Part model, mm, in its own coordinate system. Face numbers are marked on the shaded views. A direction names the side the tool comes from. Give positions to 0.01 mm unless a question says otherwise; leave off trailing zeros. Loops run counter-clockwise (first coordinate to the right, second up) from the corner with the lowest first, then second, coordinate; pieces in that order, holes last. Notation, with made-up numbers: M 45,0 L 62,0 A8 cw 62,13 Z; hole C 74.25,-36 d8. An arc over 180 degrees is marked long. Answer in a Markdown table with one row per item.
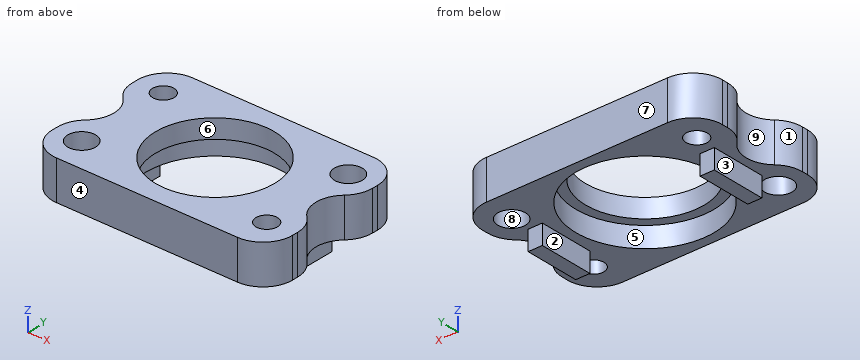
from build123d import *

# Parameters (mm, degrees)
SKETCH1_W                       = 38.735
SKETCH1_H                       = 25.4
BOSS_EXTRUDE1_DEPTH             = 6.35
CUT_EXTRUDE1_DEPTH              = 7.35
CUT_EXTRUDE2_DEPTH              = 7.35
SKETCH4_W                       = 2.286
SKETCH4_H                       = 8.89
BOSS_EXTRUDE2_DEPTH             = 3.175
SKETCH5_W                       = 2.286
SKETCH5_H                       = 8.89
BOSS_EXTRUDE3_DEPTH             = 3.175
HOLE1_D                         = 19.1262
HOLE1_DEPTH                     = 6.35
HOLE1_CBORE_D                   = 22.2758
HOLE1_CBORE_DEPTH               = 3.302
F_16_0_177_DIAMETER_HOLE1_D     = 4.4958
F_16_0_177_DIAMETER_HOLE1_DEPTH = 9.525
F_29_0_136_DIAMETER_HOLE1_D     = 3.4544
F_29_0_136_DIAMETER_HOLE1_DEPTH = 9.525
FILLET1_R                       = 4.7625


with BuildPart() as part:
    # Sketch1 → Boss-Extrude1 (new body)
    with BuildSketch(Plane.XY.offset(6.35)):
        with Locations((-234.6325, 25.4)):
            Rectangle(SKETCH1_W, SKETCH1_H)
    extrude(amount=-BOSS_EXTRUDE1_DEPTH)

    # Sketch2 → Cut-Extrude1 (cut, through all)
    with BuildSketch(Plane(origin=(0, 0, 0), x_dir=(-1, 0, 0), z_dir=(0, 0, -1))):
        with BuildLine():
            Line((215.265, 32.388210744), (215.265, 18.411789256))
            ThreePointArc((215.265, 18.411789256), (215.6632391, 20.318260617), (216.791355087, 21.905894628))
            ThreePointArc((216.791355087, 21.905894628), (218.317710174, 25.4), (216.791355087, 28.894105372))
            ThreePointArc((216.791355087, 28.894105372), (215.6632391, 30.481739383), (215.265, 32.388210744))
        make_face()
    extrude(amount=-CUT_EXTRUDE1_DEPTH, mode=Mode.SUBTRACT)

    # Sketch3 → Cut-Extrude2 (cut, through all)
    with BuildSketch(Plane(origin=(0, 0, 0), x_dir=(-1, 0, 0), z_dir=(0, 0, -1))):
        with BuildLine():
            Line((254, 20.955), (254, 29.845))
            ThreePointArc((254, 29.845), (250.969652441, 25.4), (254, 20.955))
        make_face()
    extrude(amount=-CUT_EXTRUDE2_DEPTH, mode=Mode.SUBTRACT)

    # Sketch4 → Boss-Extrude2 (add)
    with BuildSketch(Plane(origin=(0, 0, 0), x_dir=(-1, 0, 0), z_dir=(0, 0, -1))):
        with Locations((220.7641, 25.4)):
            Rectangle(SKETCH4_W, SKETCH4_H)
    extrude(amount=BOSS_EXTRUDE2_DEPTH)

    # Sketch5 → Boss-Extrude3 (add)
    with BuildSketch(Plane(origin=(0, 0, 0), x_dir=(-1, 0, 0), z_dir=(0, 0, -1))):
        with Locations((248.5009, 25.4)):
            Rectangle(SKETCH5_W, SKETCH5_H)
    extrude(amount=BOSS_EXTRUDE3_DEPTH)

    # Hole1
    with Locations(Plane(origin=(0, 0, 0), x_dir=(-1, 0, 0), z_dir=(0, 0, -1))):
        with Locations((234.6325, 25.4)):
            CounterBoreHole(HOLE1_D / 2, HOLE1_CBORE_D / 2, HOLE1_CBORE_DEPTH, depth=HOLE1_DEPTH)

    # #16 (0.177) Diameter Hole1
    with Locations(Plane.XY.offset(6.35)):
        with Locations((-249.555, 17.78), (-219.71, 33.02)):
            Hole(F_16_0_177_DIAMETER_HOLE1_D / 2, depth=F_16_0_177_DIAMETER_HOLE1_DEPTH)

    # #29 (0.136) Diameter Hole1
    with Locations(Plane.XY.offset(6.35)):
        with Locations((-219.71, 17.78), (-249.555, 33.02)):
            Hole(F_29_0_136_DIAMETER_HOLE1_D / 2, depth=F_29_0_136_DIAMETER_HOLE1_DEPTH)

    # Fillet1
    fillet1_edges = [part.edges().sort_by_distance(p)[0] for p in [
        (-254, 20.955, 3.175),
        (-254, 29.845, 3.175),
        (-254, 38.1, 3.175),
        (-215.265, 38.1, 3.175),
        (-215.265, 12.7, 3.175),
        (-254, 12.7, 3.175),
    ]]
    fillet(fillet1_edges, radius=FILLET1_R)


solid = part.part
(1) Drill centre lines: line 1 along Y through (x, z) = (-235, 3); line 2 along X through (y, z) = (27, 4.25); line 3 along Z through (x, y) = (-243.5, 35). Where is each one in solid material? Low to high.
Recorded:
| item | result |
|---|---|
| line 1 | y = 12.7 to 14.27, 36.53 to 38.1 |
| line 2 | x = -251.25 to -244.06, -225.2 to -218.04 |
| line 3 | z = 0 to 6.35 |
(2) Pin check, flat tips, straight feed: pin 1 Ø1.6 at (y, z) = (26, -1) entering from +X; pin 2 Ø1 at (y, z) = (30, 2) entering from -X; pin 3 Ø1 at (y, z) = (26, -1) entering from -X. Stop position of each tip, or through.
Recorded:
| item | result |
|---|---|
| pin 1 | stops at x = -219.62 |
| pin 2 | stops at x = -253.62 |
| pin 3 | stops at x = -249.64 |
(3) Which spindle directions (+Z, -Z, +X, -X, +Y, -Y) get a long thin tool onto all of the face, cutting with end or side? Do the marked faces 1, 2, 3, 4 and 5. Say none if no direction does.
Recorded:
| item | result |
|---|---|
| face 1 | +Z, -Z, -X |
| face 2 | -Z, +Y, -Y |
| face 3 | -Z, -X, +Y, -Y |
| face 4 | +Z, -Z, +X, -X, -Y |
| face 5 | -Z |
(4) Saw through at C-C (y = 25.4). Write the cut outline in (x, z) (3 decimals), plus the area to 3 significant figures.
Recorded:
| item | result |
|---|---|
| outline | M -250.97,0 L -249.644,0 L -249.644,-3.175 L -247.358,-3.175 L -247.358,0 L -245.77,0 L -245.77,3.302 L -244.196,3.302 L -244.196,6.35 L -250.97,6.35 Z; M -225.069,3.302 L -223.495,3.302 L -223.495,0 L -221.907,0 L -221.907,-3.175 L -219.621,-3.175 L -219.621,0 L -218.318,0 L -218.318,6.35 L -225.069,6.35 Z |
| area | 90.0 mm^2 |
(5) Pull direction X, two halves, no side cores. Call the marked faces 6, 7, 8 and 9: +X half, -X half, draft (parallel to the pull), parting line (faces both ways), or undercut.
Recorded:
| item | result |
|---|---|
| face 6 | undercut |
| face 7 | draft |
| face 8 | undercut |
| face 9 | -X half |
(6) Saw through at D-D (x = -227). Write the cut outline in (y, z), plus the area to 3 significant figures.
Recorded:
| item | result |
|---|---|
| outline | M 12.7,0 L 17.29,0 L 17.29,3.3 L 19.64,3.3 L 19.64,6.35 L 12.7,6.35 Z; M 31.16,3.3 L 33.51,3.3 L 33.51,0 L 38.1,0 L 38.1,6.35 L 31.16,6.35 Z |
| area | 72.6 mm^2 |
(7) Saw through at B-B (z = 1). Write the cut outline in (x, y) (1 decimal), plus the area to 3 significant figures.
Recorded:
| item | result |
|---|---|
| outline | M -254,17.5 A4.8 ccw -249.2,12.7 L -220,12.7 A4.8 ccw -215.3,17.5 L -215.3,18.4 A4.8 ccw -216.8,21.9 A4.8 cw -216.8,28.9 A4.8 ccw -215.3,32.4 L -215.3,33.3 A4.8 ccw -220,38.1 L -249.2,38.1 A4.8 ccw -254,33.3 L -254,32.4 A4.8 ccw -252.5,28.9 A4.8 cw -252.5,21.9 A4.8 ccw -254,18.4 Z; hole C -249.6,17.8 d4.5; hole C -249.6,33 d3.5; hole C -234.6,25.4 d22.3; hole C -219.7,33 d4.5; hole C -219.7,17.8 d3.5 |
| area | 482 mm^2 |
(8) Saw through at A-A (z = -2.25). Write the cut outline in (x, y) (3 decimals), plus the area to 3 significant figures.
Recorded:
| item | result |
|---|---|
| outline | M -249.644,20.955 L -247.358,20.955 L -247.358,29.845 L -249.644,29.845 Z; M -221.907,20.955 L -219.621,20.955 L -219.621,29.845 L -221.907,29.845 Z |
| area | 40.6 mm^2 |
